Geometry: final body of the model. Coordinates: model frame, mm. Face numbers are marked on the shaded views. A direction names the side the tool comes from. Give positions to 0.01 mm unless a question says otherwise; leave off trailing zeros. Write each loop counter-clockwise with the first axis right and the second up, starting at its lowest first coordinate (ties: lowest second). Pieces come first, ordered by that corner, then holes.
Autodesk Fusion 360 part; units mm, degrees
sketch "Sketch1" plane through (0, 0, 0) normal (0, 0, 1) x (1, 0, 0)
  line L0 (-50, 50) -> (50, 50)
  line L1 (50, 50) -> (50, -50)
  line L2 (50, -50) -> (-50, -50)
  line L3 (-50, -50) -> (-50, 50)
  line L4 (-50, 50) -> (50, -50) construction
  line L5 (50, 50) -> (-50, -50) construction
  line L6 (53, 53) -> (53, -53)
  line L7 (53, -53) -> (-53, -53)
  line L8 (-53, -53) -> (-53, 53)
  line L9 (-53, 53) -> (53, 53)
  dimension "d1" = -3
extrude "Extrude1" add sketch "Sketch1" along normal blind 35
extrude "Extrude2" add sketch "Sketch1" along normal blind 10 contours L0 L1 L2 L3
sketch "Sketch3" plane through (0, 0, 0) normal (0, 0, -1) x (1, 0, 0)
  line L0 (-53, 53) -> (-53, -53)
  line L1 (-53, -53) -> (53, -53)
  line L2 (53, -53) -> (53, 53)
  line L3 (53, 53) -> (-53, 53)
  circle A0 centre (-12.5, 0) radius 5
  circle A1 centre (12.5, 0) radius 5
  circle A2 centre (-12.5, 30) radius 5
  circle A3 centre (12.5, 30) radius 5
  circle A4 centre (-12.5, -30) radius 5
  circle A5 centre (12.5, -30) radius 5
  dimension "d6" = 10
  dimension "d7" = 10
  dimension "d8" = 25
  dimension "d9" = 12.5
  dimension "d12" = 0
  dimension "d13" = 30
  dimension "d16" = 0
  dimension "d17" = -30
extrude "Extrude3" cut sketch "Sketch3" against normal blind 10 contours A0 | A1 | A2 | A3 | A4 | A5
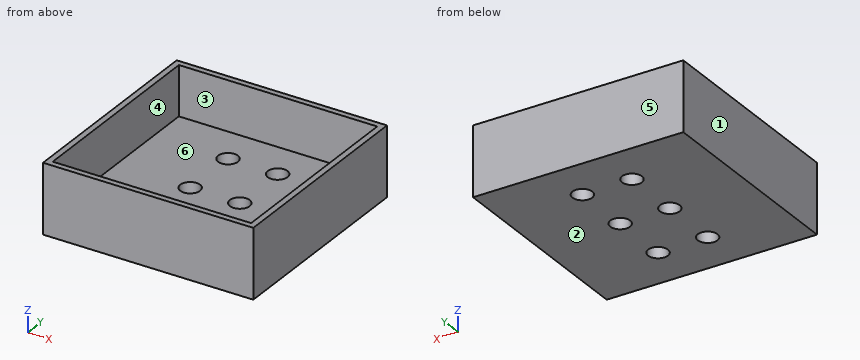
Item 1: Pull-direction query (X, two-part tool) for the marked faces 1, 2, 3 and 4; classes: +X half, -X half, draft (parallel to the pull), parting line (faces both ways), or undercut.
Found:
face 1: -X half
face 2: draft
face 3: undercut
face 4: undercut
Item 2: Section D-D, the plane x = 0. Return the cut outline in (y, z), plus the area to 3 significant figures.
Found:
outline: (-53, 0) - (53, 0) - (53, 35) - (50, 35) - (50, 10) - (-50, 10) - (-50, 35) - (-53, 35) - close
area: 1,210 mm2
Item 3: Pin query (flat end, axial travel): pin 1 Ø8 at (x, y) = (41.5, -23.5) entering from +Z. Return the tip coordinate at first contact, or that it passes through.
Found:
pin 1: stops at z = 10
Item 4: Section A-A, the plane x = 12.5. Return the cut outline in (y, z).
Found:
outline: (-53, 0) - (-35, 0) - (-35, 10) - (-50, 10) - (-50, 35) - (-53, 35) - close; (-25, 0) - (-5, 0) - (-5, 10) - (-25, 10) - close; (5, 0) - (25, 0) - (25, 10) - (5, 10) - close; (35, 0) - (53, 0) - (53, 35) - (50, 35) - (50, 10) - (35, 10) - close
Item 5: Line query: L1, parallel to X at y = 30, z = 4.25; L2, parallel to Y at x = 12, z = 4; L3, parallel to Y at x = -6, z = 32. Output: solid intervals per line, ascending.
Found:
L1: x = -53 to -17.5, -7.5 to 7.5, 17.5 to 53
L2: y = -53 to -34.97, -25.03 to -4.97, 4.97 to 25.03, 34.97 to 53
L3: y = -53 to -50, 50 to 53
Item 6: Section C-C, the plane z = 18. Return the cut outline in (x, y).
Found:
outline: (-53, -53) - (53, -53) - (53, 53) - (-53, 53) - close; hole (-50, -50) - (50, -50) - (50, 50) - (-50, 50) - close
Item 7: Reachability of the marked faces 5 and 6 from +Z, -Z, +X, -X, +Y, -Y: full face, straight path, thin tool, end or side. Return the list, or none.
Found:
face 5: +Z, -Z, +X, -X, +Y
face 6: +Z
Item 8: Section B-B, the plane y = 0. Return the cut outline in (x, z), plus the area to 3 significant figures.
Found:
outline: (-53, 0) - (-17.5, 0) - (-17.5, 10) - (-50, 10) - (-50, 35) - (-53, 35) - close; (-7.5, 0) - (7.5, 0) - (7.5, 10) - (-7.5, 10) - close; (17.5, 0) - (53, 0) - (53, 35) - (50, 35) - (50, 10) - (17.5, 10) - close
area: 1,010 mm2
